from build123d import *

# Parameters (mm, degrees)
SKETCH1_W           = 10
SKETCH1_H           = 20
BOSS_EXTRUDE1_DEPTH = 25.4
CHAMFER1_SIZE       = 10
CHAMFER1_SIZE2      = 17.320508076


with BuildPart() as part:
    # Sketch1 → Boss-Extrude1 (new body)
    with BuildSketch(Plane(origin=(0, 0, 0), x_dir=(0, 0, -1), z_dir=(1, 0, 0))):
        Rectangle(SKETCH1_W, SKETCH1_H)
    extrude(amount=BOSS_EXTRUDE1_DEPTH)

    # Chamfer1
    chamfer1_edges = [part.edges().sort_by_distance(p)[0] for p in [
        (25.4, 10, 0),
    ]]
    chamfer1_side = [part.faces().sort_by_distance(p)[0] for p in [
        (12.7, 10, 0),
    ]]
    chamfer(chamfer1_edges, length=CHAMFER1_SIZE, length2=CHAMFER1_SIZE2, reference=chamfer1_side[0])


solid = part.part
Model file for the job. Use its own axes, mm. Coordinates: 2 decimals unless noted, no trailing zeros. Order: outer loops, then holes, each group sorted by start corner. A loop starts at its lowest first (then second) coordinate and runs counter-clockwise, first axis right, second up. Notation, with made-up numbers: M 33.25,15.25 L 57.25,15.25 A24 ccw 57.25,36.25 Z; hole C -32.5,-25 d9. An arc over 180 degrees is marked long. Return JSON: item names as keys, results as strings.
1. Saw through at B-B (y = 5.75). Give the cut face in (x, z).
Ans:
{"outline": "M 0,-5 L 17.85,-5 L 17.85,5 L 0,5 Z"}
2. Flat gauge pin, fed straight in: pin 1 (1.5 mm diameter, centred on y = -4.5, z = -2.5, fed in from +X). Where does the tip first touch, or does it go through?
Ans:
{"pin 1": "x = 24.2"}
3. Drill centre lines: probe 1 along Y at (x, z) = (20.5, -0.25); probe 2 along X at (y, z) = (5.75, 3.25); probe 3 along Y at (x, z) = (19.75, 2). Where is each one in solid material? Low to high.
Ans:
{"probe 1": "-10 to 1.17", "probe 2": "0 to 17.85", "probe 3": "-10 to 2.47"}
4. Saw through at A-A (z = 0.75). Give the cut face in (x, y), and give its area (3 significant figures).
Ans:
{"outline": "M 0,-10 L 25.4,-10 L 25.4,-7.32 L 15.4,10 L 0,10 Z", "area": "421 mm^2"}
5. Saw through at C-C (x = 18.5). Give the cut face in (y, z), and give its area (3 significant figures).
Ans:
{"outline": "M -10,-5 L 4.63,-5 L 4.63,5 L -10,5 Z", "area": "146 mm^2"}
